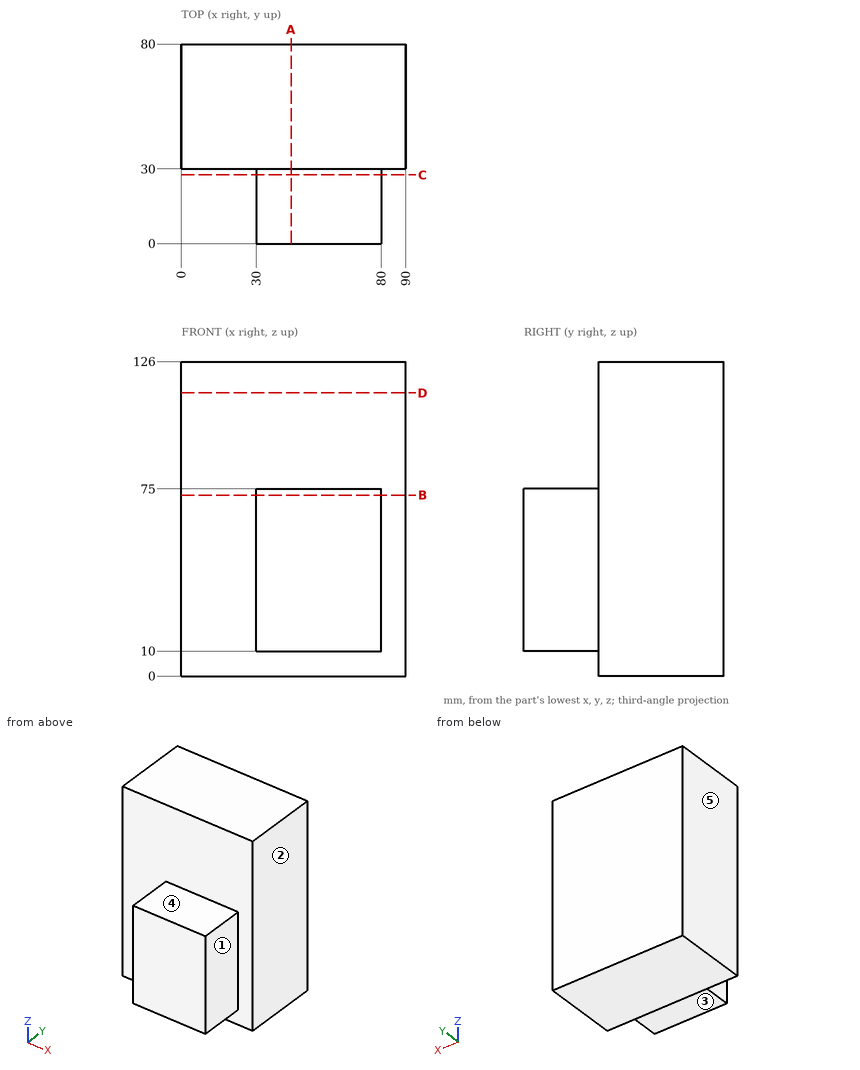
Print and shaded views of the part. All mm, measured from the part's lowest x, y and z. A direction names the side the tool comes from. Give positions to 0.01 mm unless a question says otherwise; leave off trailing zeros. Write each loop counter-clockwise with the first axis right and the second up, starting at its lowest first coordinate (ties: lowest second). Pieces come first, ordered by that corner, then holes. Notation, with made-up numbers: (-1.5, 33) -> (24.5, 33) arc R9 ccw to (24.5, 41) -> close; hole circle Ø2 at (66.5, -3). An arc over 180 degrees is marked (long way). Write item = value, one per line.
(1) Slice it at D-D, the plane z = 113.5. Give the cut face in (x, y), then the cut area to 3 significant figures.
Determined:
outline = (0, 30) -> (90, 30) -> (90, 80) -> (0, 80) -> close
area = 4,500 mm2
(2) Slice it at C-C, the plane y = 27.5. Give the cut face in (x, z).
Determined:
outline = (30, 10) -> (80, 10) -> (80, 75) -> (30, 75) -> close
(3) Slice it at A-A, the plane x = 44. Give the cut face in (y, z), then the cut area to 3 significant figures.
Determined:
outline = (0, 10) -> (30, 10) -> (30, 0) -> (80, 0) -> (80, 126) -> (30, 126) -> (30, 75) -> (0, 75) -> close
area = 8,250 mm2
(4) Flat gauge pins, fed straight in: P1, Ø2, axis at x = 72, y = 20, coming from the -Z side; P2, Ø24, axis at y = 17, z = 49, coming from the -X side; P3, Ø15, axis at y = 11, z = 49.5, coming from the +X side. Where does each tip first touch, or does it go through?
Determined:
P1 = 10
P2 = 30
P3 = 80
(5) Slice it at B-B, the plane z = 72.5. Give the cut face in (x, y).
Determined:
outline = (0, 30) -> (30, 30) -> (30, 0) -> (80, 0) -> (80, 30) -> (90, 30) -> (90, 80) -> (0, 80) -> close
(6) Tool access for the marked faces 1, 2, 3, 4 and 5: list every direction of +Z, -Z, +X, -X, +Y, -Y with a clear straight run to the whole face (end or side of a thin tool).
Determined:
face_1 = +Z, -Z, +X, -Y
face_2 = +Z, -Z, +X, +Y, -Y
face_3 = -Z, +X, -X, -Y
face_4 = +Z, +X, -X, -Y
face_5 = +Z, -Z, -X, +Y, -Y
(7) Probe line 1 along Y through (x, z) = (22.5, 78.5). List the from-to ranges inside material, lowest first.
Determined:
line_1 = 30 to 80
